Model file for the job. Use its own axes, mm. Face numbers are marked on the shaded views. A direction names the side the tool comes from. Round coordinates to 2 decimals unless told otherwise and drop trailing zeros. Loops run counter-clockwise (first coordinate to the right, second up) from the corner with the lowest first, then second, coordinate; pieces in that order, holes last. Notation, with made-up numbers: M 49.25,-24.5 L 61.25,-24.5 A36 ccw 61.25,10.5 Z; hole C 22.5,38.5 d6. An arc over 180 degrees is marked long. Use a Markdown table: item, result. Add a question column.
Item 1: Saw through at C-C on y = 27. Write the cut outline in (x, z) (3 decimals), then the cut area to 3 significant figures.
Item 2: Wall check: L1, parallel to Y at x = 21.55, z = -7.75; L2, parallel to Y at x = 20.95, z = -15.5; L3, parallel to X at y = 16.5, z = -10 (3 decimals). Give the ranges that are in metal, low to high. Write a range as from..to.
Item 3: Tool access for the marked faces 1 and 2: list every direction of +Z, -Z, +X, -X, +Y, -Y with a clear straight run to the whole face (end or side of a thin tool).
Item 4: Pin check, flat tips, straight feed: P1, Ø2, axis at y = 26.19, z = 15.5, coming from the +X side; P2, Ø4, axis at y = 39.62, z = -7.75, coming from the -X side; P3, Ø3, axis at x = -6, z = -8.5, coming from the -Y side; P4, Ø1, axis at x = 6.5, z = 9.5, coming from the +Y side (3 decimals). Stop position of each tip, or through.
Item 5: Saw through at B-B on z = 7.75. Give the number of separate pieces and of enclosed holes in the cut face, then the cut area to 3 significant figures.
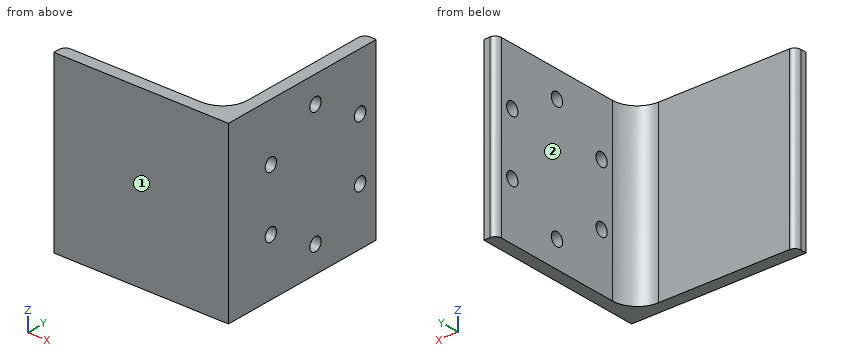
```python
from build123d import *

# Parameters (mm, degrees)
BOSS_EXTRUDE1_DEPTH  = 22.225
M3_CLEARANCE_HOLE2_D = 3.4


with BuildPart() as part:
    # Sketch2 → Boss-Extrude1 (new, symmetric)
    with BuildSketch(Plane.XY):
        with BuildLine():
            Line((-22.225, 0), (22.225, 0))
            Line((22.225, 0), (22.225, 44.45))
            Line((22.225, 44.45), (20.6375, 44.45))
            ThreePointArc((20.6375, 44.45), (19.514967985, 43.985032015), (19.05, 42.8625))
            Line((19.05, 42.8625), (19.05, 9.525))
            ThreePointArc((19.05, 9.525), (17.190128061, 5.034871939), (12.7, 3.175))
            Line((12.7, 3.175), (-20.6375, 3.175))
            ThreePointArc((-20.6375, 3.175), (-21.760032015, 2.710032015), (-22.225, 1.5875))
            Line((-22.225, 1.5875), (-22.225, 0))
        make_face()
    extrude(amount=BOSS_EXTRUDE1_DEPTH, both=True)

    # M3 Clearance Hole2 (through all)
    with Locations(Plane.ZY.offset(-19.05)):
        with Locations((7.75, 12.770356241), (15.5, 26.19375), (7.75, 39.617143759), (-7.75, 39.617143759), (-15.5, 26.19375), (-7.75, 12.770356241)):
            Hole(M3_CLEARANCE_HOLE2_D / 2)


solid = part.part
```
Entries:
| question | item | result |
|---|---|---|
| 1 | outline | M 19.05,-22.225 L 22.225,-22.225 L 22.225,-16.997 L 19.05,-16.997 Z; M 19.05,-14.003 L 22.225,-14.003 L 22.225,14.003 L 19.05,14.003 Z; M 19.05,16.997 L 22.225,16.997 L 22.225,22.225 L 19.05,22.225 Z |
| 1 | area | 122 mm2 |
| 2 | L1 | 0..11.07, 14.47..37.92, 41.32..44.45 |
| 2 | L2 | 0..24.49, 27.89..44.45 |
| 2 | L3 | 19.05..22.225 |
| 3 | face 1 | +Z, -Z, +X, -X, -Y |
| 3 | face 2 | +Z, -Z, -X, +Y |
| 4 | P1 | through |
| 4 | P2 | x = 19.05 |
| 4 | P3 | y = 0 |
| 4 | P4 | y = 3.175 |
| 5 | separate pieces | 3 |
| 5 | enclosed holes | 0 |
| 5 | area | 258 mm2 |
